from build123d import *

# Parameters (mm, degrees)
SKETCH_8_W          = 34.4
SKETCH_8_H          = 60.6
SKETCH_8_W_2        = 28.4
SKETCH_8_H_2        = 51.6
EXTRUDE_4_DEPTH     = 5
SKETCH_9_W          = 28.4
SKETCH_9_H          = 11.6
EXTRUDE_5_DEPTH     = 95
SKETCH_10_R         = 62.2
CUT_EXTRUDE_3_DEPTH = 100
SKETCH_13_W         = 38.4
SKETCH_13_H         = 64.6
SKETCH_13_W_2       = 34.4
SKETCH_13_H_2       = 60.6
EXTRUDE_7_DEPTH     = 10


with BuildPart() as part:
    # 스케치8 → 보스-돌출4 (new body)
    with BuildSketch(Plane.XY):
        with Locations((17.2, 30.3)):
            Rectangle(SKETCH_8_W, SKETCH_8_H)
        with Locations((17.2, 28.8)):
            Rectangle(SKETCH_8_W_2, SKETCH_8_H_2, mode=Mode.SUBTRACT)
    extrude(amount=-EXTRUDE_4_DEPTH)

    # 스케치9 → 보스-돌출5 (add)
    with BuildSketch(Plane.XY):
        with Locations((17.2, 8.8)):
            Rectangle(SKETCH_9_W, SKETCH_9_H)
    extrude(amount=-EXTRUDE_5_DEPTH)

    # 스케치10 → 컷-돌출3 (cut)
    with BuildSketch(Plane(origin=(0, 14.6, 0), x_dir=(1, 0, 0), z_dir=(0, 1, 0))):
        with Locations((65.2, 95)):
            Circle(SKETCH_10_R)
    extrude(amount=-CUT_EXTRUDE_3_DEPTH, mode=Mode.SUBTRACT)

    # 스케치13 → 보스-돌출7 (add)
    with BuildSketch(Plane.XY):
        with Locations((17.2, 30.3)):
            Rectangle(SKETCH_13_W, SKETCH_13_H)
        with Locations((17.2, 30.3)):
            Rectangle(SKETCH_13_W_2, SKETCH_13_H_2, mode=Mode.SUBTRACT)
    extrude(amount=-EXTRUDE_7_DEPTH)


solid = part.part
Can you work these out from the model? Positions are in its coordinate system, mm. A direction names the side the tool comes from. Give positions to 0.01 mm unless a question says otherwise; leave off trailing zeros. Write each loop counter-clockwise with the first axis right and the second up, starting at its lowest first coordinate (ties: lowest second). Pieces come first, ordered by that corner, then holes. Notation, with made-up numbers: (-29, 10) -> (-11, 10) arc R12 cw to (-11, 20) -> close; hole circle Ø6 at (-9.75, 14). An arc over 180 degrees is marked (long way). Answer as a JSON object with one key per item and string values. Group by question number.
Item 1: We'd pull the mould along Y, two halves only. Please class faces 4 (the face through (31.4, 34, -2)), 5 (the face through (17, 62.6, -5)), 6 (the face through (3, 34, -2)), 7 (the face through (-1, 30, -10)): +Y half, -Y half, draft (parallel to the pull), parting line (faces both ways), or undercut.
Item 2: Suppose I cut it at A-A (y = 19.5). Please give me the cut outline in (x, z), plus the area to 3 significant figures.
Item 3: Suppose I cut it at B-B (x = 29). Please give me the cut outline in (y, z), plus the area to 3 significant figures.
Item 4: Suppose I cut it at D-D (z = -17). Please give me the cut outline in (x, y), plus the area to 3 significant figures.
Item 5: For faces 1 (the face through (17, 54.6, -2)), 2 (the face through (34, 24, 0)), 3 (the face through (2, 35, -5)), which set-ups out of +Z, -Z, +X, -X, +Y, -Y let a thin tool reach every point of the face, with its end or its side?
Item 6: Suppose I cut it at C-C (y = 9). Please give me the cut outline in (x, z), plus the area to 3 significant figures.
Item 7: Please list where these lines run through material, in increasing order: line 1 (Y direction, x = 16, z = -6); line 2 (Y direction, x = 29.5, z = -3.5); line 3 (Y direction, x = 17, z = -33). Write a range as [from, to].
Item 8: I'm going to push flat-ended pins straight in: P1, Ø2, axis at x = 5.5, z = -39.5, coming from the +Y side; P2, Ø10.5, axis at x = 14, y = 44.5, coming from the -Z side; P3, Ø4, axis at y = 5, z = -78.5, coming from the -X side; P4, Ø19, axis at x = 10, y = 39, coming from the -Z side. Where does each tip first touch, or does it pass through?
Findings:
{
 "1": {"face 4": "undercut", "face 5": "+Y half", "face 6": "undercut", "face 7": "draft"},
 "2": {"outline": "(-2, -10) -> (0, -10) -> (0, -5) -> (3, -5) -> (3, 0) -> (-2, 0) -> close; (31.4, -5) -> (34.4, -5) -> (34.4, -10) -> (36.4, -10) -> (36.4, 0) -> (31.4, 0) -> close", "area": "70.0 mm²"},
 "3": {"outline": "(-2, -10) -> (0, -10) -> (0, -5) -> (3, -5) -> (3, -44.42) -> (14.6, -44.42) -> (14.6, 0) -> (-2, 0) -> close; (54.6, -5) -> (60.6, -5) -> (60.6, -10) -> (62.6, -10) -> (62.6, 0) -> (54.6, 0) -> close", "area": "600 mm²"},
 "4": {"outline": "(3, 3) -> (31.4, 3) -> (31.4, 14.6) -> (3, 14.6) -> close", "area": "329 mm²"},
 "5": {"face 1": "+Z, -Z", "face 2": "+Z, +X, -X, +Y, -Y", "face 3": "-Z"},
 "6": {"outline": "(-2, -10) -> (0, -10) -> (0, -5) -> (3, -5) -> (3, -95) arc R62.2 cw to (31.4, -42.79) -> (31.4, -5) -> (34.4, -5) -> (34.4, -10) -> (36.4, -10) -> (36.4, 0) -> (-2, 0) -> close", "area": "1,720 mm²"},
 "7": {"line 1": "y = [-2, 0], [3, 14.6], [60.6, 62.6]", "line 2": "y = [-2, 14.6], [54.6, 62.6]", "line 3": "y = [3, 14.6]"},
 "8": {"P1": "stops at y = 14.6", "P2": "passes through", "P3": "stops at x = 3", "P4": "stops at z = -5"}
}
